from build123d import *

# Parameters (mm, degrees)
F1_DEPTH = 2


with BuildPart() as f1:
    # F0 (on Top) → F1 (new body)
    with BuildSketch(Plane.XY):
        with BuildLine():
            ThreePointArc((0.5, 3.9283075236), (1.0177847027, 3.8269719491), (1.5175023316, 3.6577023763))
            Line((1.5175023316, 3.6577023763), (1.7091061614, 4.1195334844))
            ThreePointArc((1.7091061614, 4.1195334844), (0.871343979, 4.3740552889), (0, 4.46))
            Line((0, 4.46), (0, 3.96))
            ThreePointArc((0, 3.96), (0.2505017031, 3.9520689388), (0.5, 3.9283075236))
        make_face()
        with BuildLine():
            ThreePointArc((-0.5, 3.9283075236), (-0.2505017031, 3.9520689388), (0, 3.96))
            Line((0, 3.96), (0, 4.46))
            ThreePointArc((0, 4.46), (-0.871343979, 4.3740552889), (-1.7091061614, 4.1195334844))
            Line((-1.7091061614, 4.1195334844), (-1.5175023316, 3.6577023763))
            ThreePointArc((-1.5175023316, 3.6577023763), (-1.0177847027, 3.8269719491), (-0.5, 3.9283075236))
        make_face()
        with BuildLine():
            ThreePointArc((-0.5, 2.6024027359), (-0.2511301951, 2.6380738475), (0, 2.65))
            Line((0, 2.65), (0, 3.96))
            ThreePointArc((0, 3.96), (-0.2505017031, 3.9520689388), (-0.5, 3.9283075236))
            Line((-0.5, 3.9283075236), (-0.5, 2.6024027359))
        make_face()
        with BuildLine():
            ThreePointArc((0, 2.65), (0.2511301951, 2.6380738475), (0.5, 2.6024027359))
            Line((0.5, 2.6024027359), (0.5, 3.9283075236))
            ThreePointArc((0.5, 3.9283075236), (0.2505017031, 3.9520689388), (0, 3.96))
            Line((0, 3.96), (0, 2.65))
        make_face()
        with BuildLine():
            ThreePointArc((0, 2.15), (0.2517314161, 2.1352122363), (0.5, 2.0910523666))
            Line((0.5, 2.0910523666), (0.5, 2.6024027359))
            ThreePointArc((0.5, 2.6024027359), (0.2511301951, 2.6380738475), (0, 2.65))
            Line((0, 2.65), (0, 2.15))
        make_face()
        with BuildLine():
            ThreePointArc((-0.5, 2.0910523666), (-0.2517314161, 2.1352122363), (0, 2.15))
            Line((0, 2.15), (0, 2.65))
            ThreePointArc((0, 2.65), (-0.2511301951, 2.6380738475), (-0.5, 2.6024027359))
            Line((-0.5, 2.6024027359), (-0.5, 2.0910523666))
        make_face()
        with BuildLine():
            ThreePointArc((-0.8238964679, 1.9858737649), (-0.6640339592, 2.0448860362), (-0.5, 2.0910523666))
            Line((-0.5, 2.0910523666), (-0.5, 2.6024027359))
            ThreePointArc((-0.5, 2.6024027359), (-0.7616876954, 2.5381749063), (-1.0155002977, 2.447704873))
            Line((-1.0155002977, 2.447704873), (-0.8238964679, 1.9858737649))
        make_face()
        with BuildLine():
            ThreePointArc((0.5, 2.0910523666), (0.6640339592, 2.0448860362), (0.8238964679, 1.9858737649))
            Line((0.8238964679, 1.9858737649), (1.0155002977, 2.447704873))
            ThreePointArc((1.0155002977, 2.447704873), (0.7616876954, 2.5381749063), (0.5, 2.6024027359))
            Line((0.5, 2.6024027359), (0.5, 2.0910523666))
        make_face()
        with BuildLine():
            ThreePointArc((0.8238964679, 1.9858737649), (1.5202795796, 1.5202795796), (1.9858737649, 0.8238964679))
            Line((1.9858737649, 0.8238964679), (2.447704873, 1.0155002977))
            ThreePointArc((2.447704873, 1.0155002977), (1.8738329701, 1.8738329701), (1.0155002977, 2.447704873))
            Line((1.0155002977, 2.447704873), (0.8238964679, 1.9858737649))
        make_face()
        with BuildLine():
            ThreePointArc((-1.9858737649, 0.8238964679), (-1.5202795796, 1.5202795796), (-0.8238964679, 1.9858737649))
            Line((-0.8238964679, 1.9858737649), (-1.0155002977, 2.447704873))
            ThreePointArc((-1.0155002977, 2.447704873), (-1.8738329701, 1.8738329701), (-2.447704873, 1.0155002977))
            Line((-2.447704873, 1.0155002977), (-1.9858737649, 0.8238964679))
        make_face()
        with BuildLine():
            ThreePointArc((-2.0910523666, 0.5), (-2.0448860362, 0.6640339592), (-1.9858737649, 0.8238964679))
            Line((-1.9858737649, 0.8238964679), (-2.447704873, 1.0155002977))
            ThreePointArc((-2.447704873, 1.0155002977), (-2.5381749063, 0.7616876954), (-2.6024027359, 0.5))
            Line((-2.6024027359, 0.5), (-2.0910523666, 0.5))
        make_face()
        with BuildLine():
            Line((-2.6024027359, -0.5), (-2.0910523666, -0.5))
            ThreePointArc((-2.0910523666, -0.5), (-2.15, 0), (-2.0910523666, 0.5))
            Line((-2.0910523666, 0.5), (-2.6024027359, 0.5))
            ThreePointArc((-2.6024027359, 0.5), (-2.65, 0), (-2.6024027359, -0.5))
        make_face()
        with BuildLine():
            Line((-2.4906162885, -0.9051687706), (-2.0206886869, -0.7343822101))
            ThreePointArc((-2.0206886869, -0.7343822101), (-2.0592079492, -0.6181930297), (-2.0910523666, -0.5))
            Line((-2.0910523666, -0.5), (-2.6024027359, -0.5))
            ThreePointArc((-2.6024027359, -0.5), (-2.5545549767, -0.7048041366), (-2.4906162885, -0.9051687706))
        make_face()
        with BuildLine():
            Line((-1.0155002977, -2.447704873), (-0.8238964679, -1.9858737649))
            ThreePointArc((-0.8238964679, -1.9858737649), (-1.553857765, -1.4859428139), (-2.0206886869, -0.7343822101))
            Line((-2.0206886869, -0.7343822101), (-2.4906162885, -0.9051687706))
            ThreePointArc((-2.4906162885, -0.9051687706), (-1.9152200359, -1.8315109102), (-1.0155002977, -2.447704873))
        make_face()
        with BuildLine():
            Line((-0.5, -2.6024027359), (-0.5, -2.0910523666))
            ThreePointArc((-0.5, -2.0910523666), (-0.6640339592, -2.0448860362), (-0.8238964679, -1.9858737649))
            Line((-0.8238964679, -1.9858737649), (-1.0155002977, -2.447704873))
            ThreePointArc((-1.0155002977, -2.447704873), (-0.7616876954, -2.5381749063), (-0.5, -2.6024027359))
        make_face()
        with BuildLine():
            Line((0.5, -2.6024027359), (0.5, -2.0910523666))
            ThreePointArc((0.5, -2.0910523666), (0, -2.15), (-0.5, -2.0910523666))
            Line((-0.5, -2.0910523666), (-0.5, -2.6024027359))
            ThreePointArc((-0.5, -2.6024027359), (0, -2.65), (0.5, -2.6024027359))
        make_face()
        with BuildLine():
            Line((1.0155002977, -2.447704873), (0.8238964679, -1.9858737649))
            ThreePointArc((0.8238964679, -1.9858737649), (0.6640339592, -2.0448860362), (0.5, -2.0910523666))
            Line((0.5, -2.0910523666), (0.5, -2.6024027359))
            ThreePointArc((0.5, -2.6024027359), (0.7616876954, -2.5381749063), (1.0155002977, -2.447704873))
        make_face()
        with BuildLine():
            Line((2.447704873, -1.0155002977), (1.9858737649, -0.8238964679))
            ThreePointArc((1.9858737649, -0.8238964679), (1.5202795796, -1.5202795796), (0.8238964679, -1.9858737649))
            Line((0.8238964679, -1.9858737649), (1.0155002977, -2.447704873))
            ThreePointArc((1.0155002977, -2.447704873), (1.8738329701, -1.8738329701), (2.447704873, -1.0155002977))
        make_face()
        with BuildLine():
            Line((2.6024027359, -0.5), (2.0910523666, -0.5))
            ThreePointArc((2.0910523666, -0.5), (2.0448860362, -0.6640339592), (1.9858737649, -0.8238964679))
            Line((1.9858737649, -0.8238964679), (2.447704873, -1.0155002977))
            ThreePointArc((2.447704873, -1.0155002977), (2.5381749063, -0.7616876954), (2.6024027359, -0.5))
        make_face()
        with BuildLine():
            ThreePointArc((2.0910523666, 0.5), (2.1352122363, 0.2517314161), (2.15, 0))
            ThreePointArc((2.15, 0), (2.1352122363, -0.2517314161), (2.0910523666, -0.5))
            Line((2.0910523666, -0.5), (2.6024027359, -0.5))
            ThreePointArc((2.6024027359, -0.5), (2.6380738475, -0.2511301951), (2.65, 0))
            ThreePointArc((2.65, 0), (2.6380738475, 0.2511301951), (2.6024027359, 0.5))
            Line((2.6024027359, 0.5), (2.0910523666, 0.5))
        make_face()
        with BuildLine():
            ThreePointArc((1.9858737649, 0.8238964679), (2.0448860362, 0.6640339592), (2.0910523666, 0.5))
            Line((2.0910523666, 0.5), (2.6024027359, 0.5))
            ThreePointArc((2.6024027359, 0.5), (2.5381749063, 0.7616876954), (2.447704873, 1.0155002977))
            Line((2.447704873, 1.0155002977), (1.9858737649, 0.8238964679))
        make_face()
        with BuildLine():
            Line((3.9283075236, 0.5), (2.6024027359, 0.5))
            ThreePointArc((2.6024027359, 0.5), (2.6380738475, 0.2511301951), (2.65, 0))
            ThreePointArc((2.65, 0), (2.6380738475, -0.2511301951), (2.6024027359, -0.5))
            Line((2.6024027359, -0.5), (3.9283075236, -0.5))
            ThreePointArc((3.9283075236, -0.5), (3.9520689388, -0.2505017031), (3.96, 0))
            ThreePointArc((3.96, 0), (3.9520689388, 0.2505017031), (3.9283075236, 0.5))
        make_face()
        with BuildLine():
            ThreePointArc((3.6577023763, 1.5175023316), (3.8269719491, 1.0177847027), (3.9283075236, 0.5))
            ThreePointArc((3.9283075236, 0.5), (3.9520689388, 0.2505017031), (3.96, 0))
            ThreePointArc((3.96, 0), (3.9520689388, -0.2505017031), (3.9283075236, -0.5))
            ThreePointArc((3.9283075236, -0.5), (3.8269719491, -1.0177847027), (3.6577023763, -1.5175023316))
            Line((3.6577023763, -1.5175023316), (4.1195334844, -1.7091061614))
            ThreePointArc((4.1195334844, -1.7091061614), (4.3740552889, -0.871343979), (4.46, 0))
            ThreePointArc((4.46, 0), (4.3740552889, 0.871343979), (4.1195334844, 1.7091061614))
            Line((4.1195334844, 1.7091061614), (3.6577023763, 1.5175023316))
        make_face()
        with BuildLine():
            Line((-3.9283075236, -0.5), (-2.6024027359, -0.5))
            ThreePointArc((-2.6024027359, -0.5), (-2.65, 0), (-2.6024027359, 0.5))
            Line((-2.6024027359, 0.5), (-3.9283075236, 0.5))
            ThreePointArc((-3.9283075236, 0.5), (-3.96, 0), (-3.9283075236, -0.5))
        make_face()
        with BuildLine():
            ThreePointArc((-4.1195334844, 1.7091061614), (-4.4588872876, 0.0996200586), (-4.1917542064, -1.5234161196))
            Line((-4.1917542064, -1.5234161196), (-3.7218266048, -1.3526295591))
            ThreePointArc((-3.7218266048, -1.3526295591), (-3.8487507501, -0.9320502472), (-3.9283075236, -0.5))
            ThreePointArc((-3.9283075236, -0.5), (-3.96, 0), (-3.9283075236, 0.5))
            ThreePointArc((-3.9283075236, 0.5), (-3.8269719491, 1.0177847027), (-3.6577023763, 1.5175023316))
            Line((-3.6577023763, 1.5175023316), (-4.1195334844, 1.7091061614))
        make_face()
        with BuildLine():
            Line((0.5, -3.9283075236), (0.5, -2.6024027359))
            ThreePointArc((0.5, -2.6024027359), (0, -2.65), (-0.5, -2.6024027359))
            Line((-0.5, -2.6024027359), (-0.5, -3.9283075236))
            ThreePointArc((-0.5, -3.9283075236), (0, -3.96), (0.5, -3.9283075236))
        make_face()
        with BuildLine():
            Line((1.7091061614, -4.1195334844), (1.5175023316, -3.6577023763))
            ThreePointArc((1.5175023316, -3.6577023763), (1.0177847027, -3.8269719491), (0.5, -3.9283075236))
            ThreePointArc((0.5, -3.9283075236), (0, -3.96), (-0.5, -3.9283075236))
            ThreePointArc((-0.5, -3.9283075236), (-1.0177847027, -3.8269719491), (-1.5175023316, -3.6577023763))
            Line((-1.5175023316, -3.6577023763), (-1.7091061614, -4.1195334844))
            ThreePointArc((-1.7091061614, -4.1195334844), (0, -4.46), (1.7091061614, -4.1195334844))
        make_face()
    extrude(amount=F1_DEPTH)


solid = f1.part
Work out the finished part from the listing and answer in its coordinate system (mm). Give positions to 0.01 mm unless a question says otherwise; leave off trailing zeros. Write each loop counter-clockwise with the first axis right and the second up, starting at its lowest first coordinate (ties: lowest second). Pieces come first, ordered by that corner, then holes.
Q1. Given pin 1 (0.7 mm diameter, centred on y = -3, z = 1, fed in from +X); pin 2 (1 mm diameter, centred on x = 1, z = 2, fed in from -Y), each flat-ended and moving along its own axis, determine where each tip first touches the part or whether it passes through.
Answer:
pin 1: stops at x = 0.5
pin 2: stops at y = -4.43
Q2. Straight lines are drawn through the part: L1, parallel to X at y = -1, z = 0.9; L2, parallel to Y at x = -0.75, z = 1.8. For each, find the intervals that lie inside material, in ascending order.
Answer:
L1: x = -4.35 to -3.83, -2.45 to -1.9, 1.9 to 2.45, 3.83 to 4.35
L2: y = -4.4 to -3.89, -2.54 to -2.01, 2.01 to 2.54, 3.89 to 4.4
Q3. The part is cut by section A-A on y = -3.5. Give the vertices of the cut face in (x, z).
Answer:
outline: (-0.5, 0) - (0.5, 0) - (0.5, 2) - (-0.5, 2) - close
Q4. For a pull along X with two mould halves and no side action, classify faces 1 (the face through (-3, -0.5, 1)), 2 (the face through (-4.46, 0.12, 0.99)), 3 (the face through (1.6, 1.7, 0)) as released by +X, released by -X, zero draft, split by the parting line, or undercut.
Answer:
face 1: undercut
face 2: released by -X
face 3: zero draft
